from build123d import *

# Parameters (mm, degrees)
F0_R     = 7.75
F0_R_2   = 6.25
F1_DEPTH = 32.3
F2_R     = 1.25
F3_DEPTH = 12.5


with BuildPart() as f1:
    # F0 (on Right) → F1 (new body, symmetric)
    with BuildSketch(Plane.YZ):
        Circle(F0_R)
        Circle(F0_R_2, mode=Mode.SUBTRACT)
    extrude(amount=F1_DEPTH, both=True)

    # F2 (on Front) → F3 (cut, symmetric)
    with BuildSketch(Plane.XZ):
        with Locations((-29.5, 0)):
            Circle(F2_R)
        with Locations((29.5, 0)):
            Circle(F2_R)
    extrude(amount=F3_DEPTH, both=True, mode=Mode.SUBTRACT)


solid = f1.part
Work out the finished part from the listing and answer in its coordinate system (mm). Give positions to 0.01 mm unless a question says otherwise; leave off trailing zeros. Order: outer loops, then holes, each group sorted by start corner. A loop starts at its lowest first (then second) coordinate and runs counter-clockwise, first axis right, second up. Notation, with made-up numbers: (-33, -2.75) - (-28, -2.75) arc R23 cw to (-28, 13.25) - close; hole circle Ø8 at (43, -14.75). An arc over 180 degrees is marked (long way). Answer as CSV lines item,"result". Start each with the question number.
Q1. The mould has two halves that part along Z. Classify faces 1 (the face through (-32.3, 0.5, 6.4)), 2 (the face through (-29.66, 6.93, 1.24)), 3 (the face through (0.5, 7.4, 2.3)): +Z half, -Z half, draft (parallel to the pull), parting line (faces both ways), or undercut.
Q2. The part is cut by section B-B (x = 29.5). Write down the section's boundary in (y, z), then the cut area to 3 significant figures.
Q3. Find the intervals of material crossed by L1, parallel to X at y = 7.05, z = 0; L2, parallel to Z at x = 27.5, y = 0, in increasing order. Write a range as [from, to].
Q4. The part is cut by section A-A (y = 0). Write down the section's boundary in (x, z).
Q5. Given pin 1 Ø5 at (x, y) = (9.5, 5.5) entering from -Z; pin 2 Ø2 at (x, z) = (29.5, 0) entering from +Y; pin 3 Ø6 at (x, y) = (3, -4.5) entering from +Z; pin 4 Ø1.5 at (x, z) = (13, 3) entering from -Y, each flat-ended and moving along its own axis, determine where each tip first touches the part or whether it passes through.
Q6. The part is cut by section C-C (x = -27). Write down the section's boundary in (y, z).
Check result:
1,face 1,"draft"
1,face 2,"undercut"
1,face 3,"parting line"
2,outline,"(-7.65, -1.25) arc R7.75 ccw to (7.65, -1.25) - (6.12, -1.25) arc R6.25 cw to (-6.12, -1.25) - close; (-7.65, 1.25) - (-6.12, 1.25) arc R6.25 cw to (6.12, 1.25) - (7.65, 1.25) arc R7.75 ccw to start"
2,area,"58.4 mm²"
3,L1,"x = [-32.3, -30.75], [-28.25, 28.25], [30.75, 32.3]"
3,L2,"z = [-7.75, -6.25], [6.25, 7.75]"
4,outline,"(-32.3, -7.75) - (32.3, -7.75) - (32.3, -6.25) - (-32.3, -6.25) - close; (-32.3, 6.25) - (32.3, 6.25) - (32.3, 7.75) - (-32.3, 7.75) - close"
5,pin 1,"stops at z = -7.15"
5,pin 2,"passes through"
5,pin 3,"stops at z = 7.6"
5,pin 4,"stops at y = -7.42"
6,outline,"circle Ø15.5 at (0, 0); hole circle Ø12.5 at (0, 0)"
